Job drawing, mm, ordinate dimensions from the low corner. One solid piece. A direction names the side the tool comes from. Round coordinates to 2 decimals unless told otherwise and drop trailing zeros. Write each loop counter-clockwise with the first axis right and the second up, starting at its lowest first coordinate (ties: lowest second). Pieces come first, ordered by that corner, then holes.
1) Saw through at B-B on y = 9. Write the cut outline in (x, z).
2) Drill centre lines: L1, parallel to Z at x = 15.75, y = 14.5; L2, parallel to Y at x = 16.25, z = 30; L3, parallel to Y at x = 13, z = 29 (1 decimal). Where is each one in solid material? Low to high.
3) Which spindle directions (+Z, -Z, +X, -X, +Y, -Y) get a long thin tool onto all of the face, cutting with end or side? Do the marked faces 1, 2 and 3. Say none if no direction does.
4) Pull direction Z, two halves, no side cores. Call the marked faces 4, 5 and 6: +Z half, -Z half, draft (parallel to the pull), parting line (faces both ways), or undercut.
5) Saw through at C-C on z = 44. Write the cut outline in (x, y).
6) Flat gauge pins, fed straight in: pin 1 (6.5 mm diameter, centred on y = 25.5, z = 20.47, fed in from -X); pin 2 (10 mm diameter, centred on x = 7.5, y = 28.5, fed in from +Z); pin 3 (1.5 mm diameter, centred on x = 5.5, y = 1.5, fed in from -Z). Where does each tip first touch, or does it go through?
7) Saw through at A-A on z = 5. Write the cut outline in (x, y), and give its area (3 significant figures).
8) Saw through at D-D on z = 31. Count the separate pieces of the cut face and the enclosed holes in it.
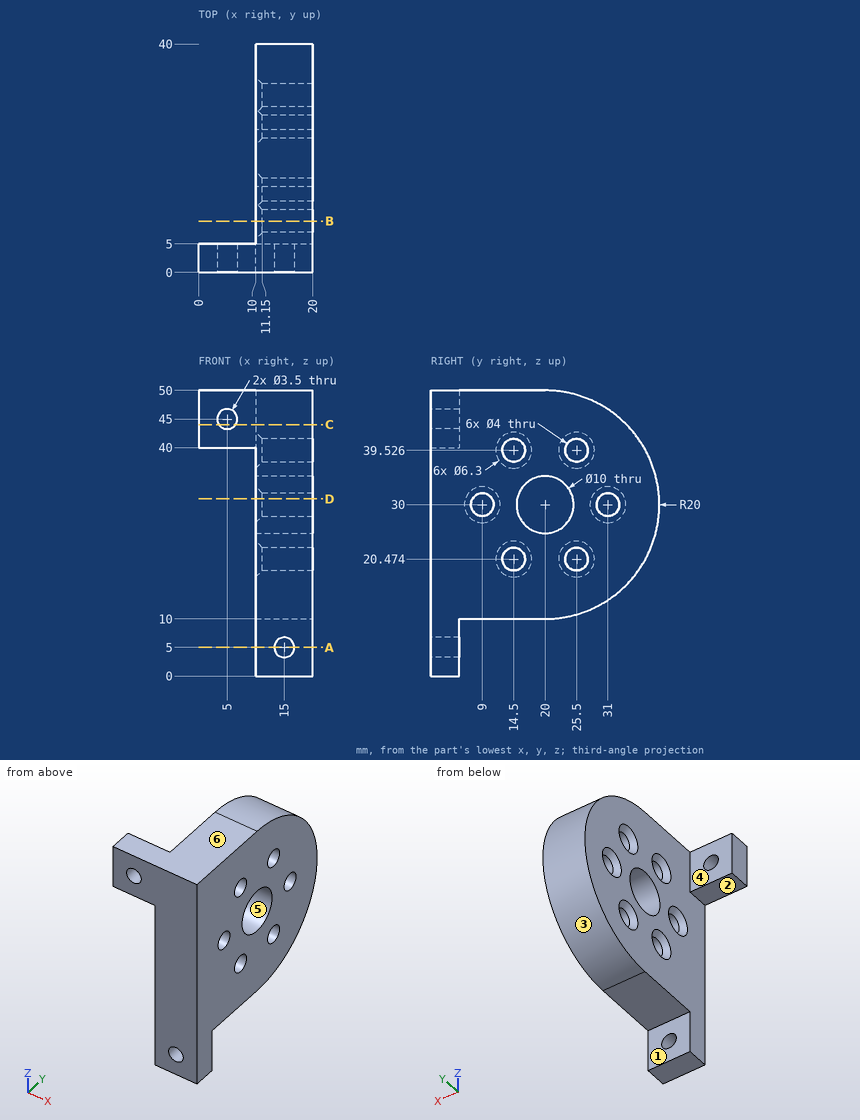
Completed:
1. outline: (10, 10) - (20, 10) - (20, 28) - (11.15, 28) - (10, 26.85) - close; (10, 33.15) - (11.15, 32) - (20, 32) - (20, 50) - (10, 50) - close
2. L1: z = 10 to 18.47, 22.47 to 37.53, 41.53 to 50
2. L2: y = 0 to 7, 11 to 15, 25 to 29, 33 to 40
2. L3: y = 0 to 7.3, 10.7 to 15.1, 24.9 to 29.3, 32.7 to 40
3. face 1: -Z, +X, -X, +Y
3. face 2: -Z, -X, +Y, -Y
3. face 3: +X, -X, +Y
4. face 4: draft
4. face 5: undercut
4. face 6: +Z half
5. outline: (0, 0) - (3.56, 0) - (3.56, 5) - (0, 5) - close; (6.44, 0) - (20, 0) - (20, 34.28) - (10, 34.28) - (10, 5) - (6.44, 5) - close
6. pin 1: stops at x = 10
6. pin 2: stops at z = 49.56
6. pin 3: stops at z = 40
7. outline: (10, 0) - (13.25, 0) - (13.25, 5) - (10, 5) - close; (16.75, 0) - (20, 0) - (20, 5) - (16.75, 5) - close
7. area: 32.5 mm2
8. separate pieces: 4
8. enclosed holes: 0
